Check sheet for the modelled part. Datum: model origin and axes. Units: mm. A direction names the side the tool comes from. Coordinates: 2 decimals unless noted, no trailing zeros. Write each loop counter-clockwise with the first axis right and the second up, starting at its lowest first coordinate (ties: lowest second). Pieces come first, ordered by that corner, then holes. Notation, with made-up numbers: (-30, -20.75) -> (2, -20.75) arc R24 ccw to (2, -7.75) -> close; hole circle Ø7 at (3, 12.25). An arc over 180 degrees is marked (long way). Put each result on its own line as item: value.
```python
from build123d import *

# Parameters (mm, degrees)
RESSALTO_EXTRUS_O1_DEPTH                            = 3
ESBO_O2_W                                           = 60.6
ESBO_O2_H                                           = 115
RESSALTO_EXTRUS_O2_DEPTH                            = 3
RESSALTO_EXTRUS_O3_DEPTH                            = 3
REBAIXO_PARA_SHCS_M21_D                             = 2.4
REBAIXO_PARA_SHCS_M21_DEPTH                         = 3
REBAIXO_PARA_SHCS_M21_CBORE_D                       = 4.4
REBAIXO_PARA_SHCS_M21_CBORE_DEPTH                   = 2
PADR_OCIRCULAR1_COUNT                               = 5
PADR_OCIRCULAR1_ANGLE                               = 180
NERVURA1_REACH                                      = 114.814
ESBO_O6_WALL_W                                      = 237.528305154
ESBO_O6_WALL_H                                      = 15
CORTE_EXTRUS_O1_REACH                               = 117.612
ESBO_O7_W                                           = 10
ESBO_O7_H                                           = 7
NERVURA7_REACH                                      = 114.814
ESBO_O8_WALL_W                                      = 237.528305154
ESBO_O8_WALL_H                                      = 15
CORTE_EXTRUS_O2_REACH                               = 114.814
ESBO_O9_W                                           = 10
ESBO_O9_H                                           = 7
PADR_O_LINEAR1_COUNT                                = 2
PADR_O_LINEAR1_PITCH                                = 84.45
ESBO_O10_R                                          = 2.75
RESSALTO_EXTRUS_O4_DEPTH                            = 0.6
REBAIXO_PARA_PARAFUSO_COM_CABE_A_PANELA_D           = 3.4
REBAIXO_PARA_PARAFUSO_COM_CABE_A_PANELA_CBORE_D     = 7
REBAIXO_PARA_PARAFUSO_COM_CABE_A_PANELA_CBORE_DEPTH = 1.5


with BuildPart() as part:
    # Esboço1 → Ressalto-extrusão1 (new body)
    with BuildSketch(Plane.XY):
        with BuildLine():
            Line((11, 0), (11, 25))
            Line((11, 25), (-11, 25))
            Line((-11, 25), (-11, 0))
            ThreePointArc((-11, 0), (-7.75, -3.25), (-4.5, 0))
            ThreePointArc((-4.5, 0), (0, 4.5), (4.5, 0))
            ThreePointArc((4.5, 0), (7.75, -3.25), (11, 0))
        make_face()
    extrude(amount=RESSALTO_EXTRUS_O1_DEPTH)

    # Esboço2 → Ressalto-extrusão2 (add)
    with BuildSketch(Plane(origin=(0, 25, 0), x_dir=(1, 0, 0), z_dir=(0, 1, 0))):
        with Locations((0, 47.5)):
            Rectangle(ESBO_O2_W, ESBO_O2_H)
    extrude(amount=RESSALTO_EXTRUS_O2_DEPTH)

    # Esboço3 → Ressalto-extrusão3 (add)
    with BuildSketch(Plane(origin=(0, 0, -81.45), x_dir=(-1, 0, 0), z_dir=(0, 0, -1))):
        with BuildLine():
            Line((-11, 0), (-11, 25))
            Line((-11, 25), (11, 25))
            Line((11, 25), (11, 0))
            ThreePointArc((11, 0), (0, -11), (-11, 0))
        make_face()
    extrude(amount=RESSALTO_EXTRUS_O3_DEPTH)

    # Rebaixo para SHCS M21
    with Locations(Plane.XY.offset(3)):
        with Locations((8, 0)):
            rebaixo_para_shcs_m21 = CounterBoreHole(REBAIXO_PARA_SHCS_M21_D / 2, REBAIXO_PARA_SHCS_M21_CBORE_D / 2, REBAIXO_PARA_SHCS_M21_CBORE_DEPTH, depth=REBAIXO_PARA_SHCS_M21_DEPTH)

    # PadrãoCircular1: Rebaixo para SHCS M21 ×5 about axis
    padr_ocircular1_axis = Axis((0, 0, 0), (0, 0, 1))
    for i in range(1, PADR_OCIRCULAR1_COUNT):
        add(rebaixo_para_shcs_m21.rotate(padr_ocircular1_axis, i * PADR_OCIRCULAR1_ANGLE / (PADR_OCIRCULAR1_COUNT - 1)), mode=Mode.SUBTRACT)

    # Esboço6 wall → Nervura1 (add, up to next)
    with BuildSketch(Plane(origin=(0, 21.5, 6.5), x_dir=(0, 0.707106781187, 0.707106781187), z_dir=(0, -0.707106781187, 0.707106781187)), mode=Mode.PRIVATE) as nervura1_sk1:
        Rectangle(ESBO_O6_WALL_W, ESBO_O6_WALL_H)
    nervura1_tool1 = extrude(nervura1_sk1.sketch, amount=-NERVURA1_REACH, mode=Mode.PRIVATE) - part.part
    nervura1 = nervura1_tool1.solids().sort_by_distance((0, 21.5, 6.5))[0]
    add(nervura1)

    # Corte-extrusão1: up to this face of the body (flat: up to its plane)
    corte_extrus_o1_end = Plane(part.part.faces().sort_by_distance((0, 21.5, 6.5))[0])
    # Esboço7 → Corte-extrusão1 (cut, up to the picked face)
    with BuildSketch(Plane.XY.offset(3), mode=Mode.PRIVATE) as corte_extrus_o1_sk1:
        with Locations((0, 21.5)):
            Rectangle(ESBO_O7_W, ESBO_O7_H)
    corte_extrus_o1_tool1 = split(extrude(corte_extrus_o1_sk1.sketch, amount=CORTE_EXTRUS_O1_REACH, mode=Mode.PRIVATE), bisect_by=corte_extrus_o1_end, keep=Keep.BOTH, mode=Mode.PRIVATE)
    corte_extrus_o1 = corte_extrus_o1_tool1.solids().sort_by(Axis((0, 21.5, 3), (0, 0, 1)))[0]
    add(corte_extrus_o1, mode=Mode.SUBTRACT)

    # Esboço8 wall → Nervura7 (add, up to next)
    with BuildSketch(Plane(origin=(0, 21.5, -3.5), x_dir=(0, 0.707106781187, -0.707106781187), z_dir=(0, 0.707106781187, 0.707106781187)), mode=Mode.PRIVATE) as nervura7_sk1:
        Rectangle(ESBO_O8_WALL_W, ESBO_O8_WALL_H)
    nervura7_tool1 = extrude(nervura7_sk1.sketch, amount=NERVURA7_REACH, mode=Mode.PRIVATE) - part.part
    nervura7 = nervura7_tool1.solids().sort_by_distance((0, 21.5, -3.5))[0]
    add(nervura7)

    # Corte-extrusão2: up to this face of the body (flat: up to its plane)
    corte_extrus_o2_end = Plane(part.part.faces().sort_by_distance((0, 21.5, -3.5))[0])
    # Esboço9 → Corte-extrusão2 (cut, up to the picked face)
    with BuildSketch(Plane(origin=(0, 0, 0), x_dir=(-1, 0, 0), z_dir=(0, 0, -1)), mode=Mode.PRIVATE) as corte_extrus_o2_sk1:
        with Locations((0, 21.5)):
            Rectangle(ESBO_O9_W, ESBO_O9_H)
    corte_extrus_o2_tool1 = split(extrude(corte_extrus_o2_sk1.sketch, amount=CORTE_EXTRUS_O2_REACH, mode=Mode.PRIVATE), bisect_by=corte_extrus_o2_end, keep=Keep.BOTH, mode=Mode.PRIVATE)
    corte_extrus_o2 = corte_extrus_o2_tool1.solids().sort_by(Axis((0, 21.5, 0), (0, 0, -1)))[0]
    add(corte_extrus_o2, mode=Mode.SUBTRACT)

    # Padrão linear1: Nervura1, Corte-extrusão1, Nervura7, Corte-extrusão2 ×2
    with Locations(*[(0, 0, -i * PADR_O_LINEAR1_PITCH) for i in range(1, PADR_O_LINEAR1_COUNT)]):
        add(nervura1)
        add(corte_extrus_o1, mode=Mode.SUBTRACT)
        add(nervura7)
        add(corte_extrus_o2, mode=Mode.SUBTRACT)

    # Esboço10 → Ressalto-extrusão4 (add)
    with BuildSketch(Plane.XY.offset(-81.45)):
        with Locations(Location((0, 0, 0), (0, 0, 180))):
            Circle(ESBO_O10_R)
    extrude(amount=RESSALTO_EXTRUS_O4_DEPTH)

    # Rebaixo para parafuso com cabeça panela de M31 (through all)
    with Locations(Plane(origin=(0, 0, -84.45), x_dir=(-1, 0, 0), z_dir=(0, 0, -1))):
        with Locations((0, 0)):
            CounterBoreHole(REBAIXO_PARA_PARAFUSO_COM_CABE_A_PANELA_D / 2, REBAIXO_PARA_PARAFUSO_COM_CABE_A_PANELA_CBORE_D / 2, REBAIXO_PARA_PARAFUSO_COM_CABE_A_PANELA_CBORE_DEPTH)


solid = part.part
```
Q1. Cross-section at C-C (z = -88). Record the cut outline in (x, y).
Recorded:
outline: (-30.3, 25) -> (-7.5, 25) -> (-7.5, 21.55) -> (-5, 21.55) -> (-5, 25) -> (5, 25) -> (5, 21.55) -> (7.5, 21.55) -> (7.5, 25) -> (30.3, 25) -> (30.3, 28) -> (-30.3, 28) -> close
Q2. Material ranges on line 1 along Y through (x, z) = (8, 0.5); line 2 along Y through (x, z) = (0, -84); line 3 along Z through (x, y) = (10.5, 10.5), recorded low to high.
Recorded:
line 1: y = -3.24 to -1.2, 1.2 to 28
line 2: y = -11 to -3.5, 3.5 to 28
line 3: z = -84.45 to -81.45, 0 to 3
Q3. Depth check by flat-ended pin: P1, Ø1.5, axis at x = -9, y = 15, coming from the +Z side; P2, Ø5, axis at y = 20, z = -83.5, coming from the +X side; P3, Ø6, axis at x = 1.5, z = -44.5, coming from the -Y side. Enter the tip coordinate at first touch or a pass-through.
Recorded:
P1: stops at z = 3
P2: stops at x = 11
P3: stops at y = 25
Q4. Tool access check on faces 1 (the cylindrical face through (-7.805, 5.181, 2.014)), 2 (the flat face through (6, 21, -3)), 3 (the flat face through (0, 25, 6)), 4 (the flat face through (-11, 13, -83)), 5 (the flat face through (-5, 23, -80)). Record the directions out of +Z, -Z, +X, -X, +Y, -Y that give a thin tool (end or side, any length) a straight path to the whole face; none if there is none.
Recorded:
face 1: +Z
face 2: +X, -X, -Y
face 3: +Z, -Y
face 4: +Z, -Z, -X, -Y
face 5: -Y
Q5. Cross-section at D-D (z = -11). Record the cut outline in (x, y), plus the area to 3 significant figures.
Recorded:
outline: (-30.3, 25) -> (30.3, 25) -> (30.3, 28) -> (-30.3, 28) -> close
area: 182 mm2
Q6. Cross-section at A-A (x = 0). State how many separate pieces and enclosed holes the cut face has, plus the area to 3 significant figures.
Recorded:
separate pieces: 3
enclosed holes: 0
area: 489 mm2
Q7. Cross-section at B-B (y = 12). Record the cut outline in (x, z).
Recorded:
outline: (-11, -84.45) -> (11, -84.45) -> (11, -81.45) -> (-11, -81.45) -> close; (-11, 0) -> (11, 0) -> (11, 3) -> (-11, 3) -> close
Q8. Mould release check, pull along Z, two halves, no side actions. Record for faces 6 (the flat face through (-5, 23, -2)), 7 (the flat face through (0, 26, -105)), 8 (the flat face through (-11, 13, 1)): released by +Z, released by -Z, zero draft, split by the parting line, or undercut.
Recorded:
face 6: undercut
face 7: released by -Z
face 8: zero draft
